The model under review builds one solid part; all positions refer to its coordinate system, in mm. Face numbers are marked on the shaded views. A direction names the side the tool comes from. Coordinates: 2 decimals unless noted, no trailing zeros. Order: outer loops, then holes, each group sorted by start corner. A loop starts at its lowest first (then second) coordinate and runs counter-clockwise, first axis right, second up. Notation, with made-up numbers: (79.25, -33.75) -> (109.25, -33.75) arc R24 ccw to (109.25, -19.75) -> close; hole circle Ø3 at (52.5, -25.5). An arc over 180 degrees is marked (long way). Use one line per item in the form item = value.
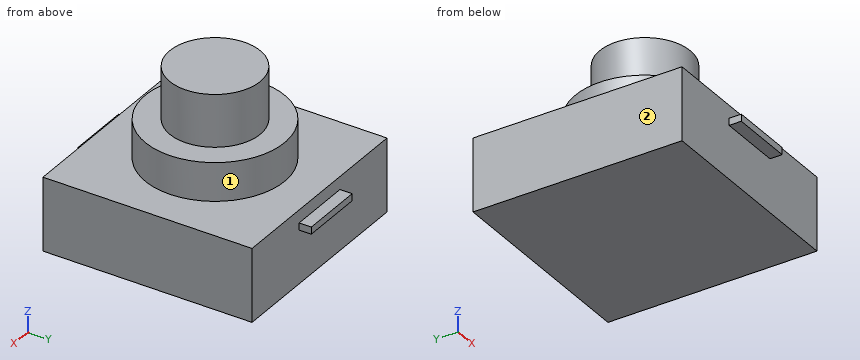
from build123d import *

# Parameters (mm, degrees)
F0_W     = 12
F0_H     = 12
F1_DEPTH = 4.2
F2_R     = 4
F3_DEPTH = 2.2
F4_R     = 2.6
F5_DEPTH = 3
F6_W     = 3.6317317281
F6_H     = 0.4035253078
F7_DEPTH = 0.7


# Not quite as in the source:
# - a pattern or mirror of a feature is missing from the dataset's text; its kind, count and spacing are read off the source's solid


with BuildPart() as f1:
    # F0 (on Top) → F1 (new body)
    with BuildSketch(Plane.XY):
        Rectangle(F0_W, F0_H)
    extrude(amount=F1_DEPTH)

    # F2 (on face) → F3 (join)
    with BuildSketch(Plane.XY.offset(4.2)):
        Circle(F2_R)
    extrude(amount=F3_DEPTH)

    # F4 (on face) → F5 (join)
    with BuildSketch(Plane.XY.offset(6.4)):
        Circle(F4_R)
    extrude(amount=F5_DEPTH)

    # F6 (on face) → F7 (join)
    with BuildSketch(Plane(origin=(0, 6, 0), x_dir=(-1, 0, 0), z_dir=(0, 1, 0))):
        with Locations((0, 3.2601370476)):
            Rectangle(F6_W, F6_H)
    f7 = extrude(amount=F7_DEPTH)

    # F7_copies: F7 across plane
    add(f7.mirror(Plane(origin=(0, 0, 0), x_dir=(0, 0, -1), z_dir=(0, -1, 0))))


solid = f1.part
Item 1: To check wall thickness, follow L1, parallel to Z at x = -1.75, y = 2.25; L2, parallel to Z at x = 4, y = 2; L3, parallel to Y at x = 1.25, z = 3.5. State the ranges of each line that lie inside material, in increasing order. Write a range as from..to.
Results found:
L1 = 0..6.4
L2 = 0..4.2
L3 = -6..6
Item 2: We need section B-B (x = 0). Write out the cut boundary in (y, z), plus the area to 3 significant figures.
Results found:
outline = (-6.7, 3.06) -> (-6, 3.06) -> (-6, 0) -> (6, 0) -> (6, 3.06) -> (6.7, 3.06) -> (6.7, 3.46) -> (6, 3.46) -> (6, 4.2) -> (4, 4.2) -> (4, 6.4) -> (2.6, 6.4) -> (2.6, 9.4) -> (-2.6, 9.4) -> (-2.6, 6.4) -> (-4, 6.4) -> (-4, 4.2) -> (-6, 4.2) -> (-6, 3.46) -> (-6.7, 3.46) -> close
area = 84.2 mm²
Item 3: Clearance check with flat-ended pins moving along their axes: pin 1 (2 mm diameter, centred on x = -4.5, z = 3, fed in from -Y); pin 2 (5 mm diameter, centred on x = -0.5, z = 7.5, fed in from -Y); pin 3 (0.6 mm diameter, centred on x = -0.5, y = 6.5, fed in from +Z). State where each tip first meets the part, or that it passes through.
Results found:
pin_1 = -6
pin_2 = -4
pin_3 = 3.46
Item 4: We need section A-A (y = 0). Write out the cut boundary in (x, z).
Results found:
outline = (-6, 0) -> (6, 0) -> (6, 4.2) -> (4, 4.2) -> (4, 6.4) -> (2.6, 6.4) -> (2.6, 9.4) -> (-2.6, 9.4) -> (-2.6, 6.4) -> (-4, 6.4) -> (-4, 4.2) -> (-6, 4.2) -> close
Item 5: We need section C-C (z = 7.5). Write out the cut boundary in (x, y).
Results found:
outline = circle Ø5.2 at (0, 0)
Item 6: Tool access review of the marked faces 1 and 2: name each direction out of +Z, -Z, +X, -X, +Y, -Y from which nothing blocks a thin tool from reaching the whole face with its end or side.
Results found:
face_1 = +Z
face_2 = +Z, -Z, -X, +Y, -Y
Item 7: We need section D-D (x = -3.5). Write out the cut boundary in (y, z), plus the area to 3 significant figures.
Results found:
outline = (-6, 0) -> (6, 0) -> (6, 4.2) -> (1.94, 4.2) -> (1.94, 6.4) -> (-1.94, 6.4) -> (-1.94, 4.2) -> (-6, 4.2) -> close
area = 58.9 mm²
